Build history of the part. All positions in model axes, mm. Face numbers are marked on the shaded views. Give positions to 0.01 mm unless a question says otherwise; leave off trailing zeros. Order: outer loops, then holes, each group sorted by start corner. A loop starts at its lowest first (then second) coordinate and runs counter-clockwise, first axis right, second up. Notation, with made-up numbers: M -22,67.5 L -17,67.5 A9 ccw -17,77.5 Z; hole C 53,25 d5. An arc over 180 degrees is marked long. One line per item, written item: value.
from build123d import *

# Parameters (mm, degrees)
BOSS_EXTRUDE1_START      = -1
SKETCH1_W                = 40
SKETCH1_H                = 10
BOSS_EXTRUDE1_DEPTH      = 5
BOSS_EXTRUDE2_DEPTH      = 5
BOSS_EXTRUDE2_DEPTH_BACK = 5
SKETCH3_W                = 10
SKETCH3_H                = 10
BOSS_EXTRUDE3_DEPTH      = 5
FILLET1_R                = 3
FILLET2_R                = 3
FILLET3_R                = 0.5
FILLET4_R                = 10
CUT_EXTRUDE1_DEPTH       = 25.669870287
CUT_EXTRUDE1_DEPTH_BACK  = 25.669870287
SKETCH4_R                = 1.875
CUT_EXTRUDE2_START       = 5
SKETCH5_R                = 3.5
CUT_EXTRUDE2_DEPTH       = 10
SKETCH7_W                = 51.703075982
SKETCH7_H                = 23.04476915
CUT_EXTRUDE4_DEPTH       = 25.669870308


with BuildPart() as part:
    # Sketch1 → Boss-Extrude1 (new body)
    with BuildSketch(Plane(origin=(0, 0, 0), x_dir=(1, 0, 0), z_dir=(0, 1, 0)).offset(BOSS_EXTRUDE1_START)):
        Rectangle(SKETCH1_W, SKETCH1_H)
    extrude(amount=-BOSS_EXTRUDE1_DEPTH)

    # Fillet2
    fillet2_edges = [part.edges().sort_by_distance(p)[0] for p in [
        (20, -3.5, 5),
        (-20, -3.5, 5),
        (-20, -3.5, -5),
        (20, -3.5, -5),
    ]]
    fillet(fillet2_edges, radius=FILLET2_R)


with BuildPart() as body_2:
    # Sketch2 → Boss-Extrude2 (new, two sides: drawn at the far end of the back side and taken through both)
    with BuildSketch(Plane.XY.offset(-BOSS_EXTRUDE2_DEPTH_BACK)):
        with BuildLine():
            Line((-10.378945033, 0), (-4.733920151, 0))
            ThreePointArc((-4.733920151, 0), (0, 8.3), (4.733920151, 0))
            Line((4.733920151, 0), (10.378945033, 0))
            ThreePointArc((10.378945033, 0), (0, 13.55), (-10.378945033, 0))
        make_face()
    extrude(amount=BOSS_EXTRUDE2_DEPTH + BOSS_EXTRUDE2_DEPTH_BACK)

    # Sketch3 → Boss-Extrude3 (add)
    with BuildSketch(Plane(origin=(0, 0, 0), x_dir=(1, 0, 0), z_dir=(0, 1, 0))):
        with Locations((-15, 0)):
            Rectangle(SKETCH3_W, SKETCH3_H)
        with Locations((15, 0)):
            Rectangle(SKETCH3_W, SKETCH3_H)
    extrude(amount=BOSS_EXTRUDE3_DEPTH)

    # Fillet1
    fillet1_edges = [body_2.edges().sort_by_distance(p)[0] for p in [
        (-20, 2.5, -5),
        (-20, 2.5, 5),
        (20, 2.5, 5),
        (20, 2.5, -5),
    ]]
    fillet(fillet1_edges, radius=FILLET1_R)

    # Fillet3
    fillet3_edges = [body_2.edges().sort_by_distance(p)[0] for p in [
        (-4.733920151, 0, 0),
        (4.733920151, 0, 0),
    ]]
    fillet(fillet3_edges, radius=FILLET3_R)

    # Fillet4
    fillet4_edges = [body_2.edges().sort_by_distance(p)[0] for p in [
        (-10.522475944, 5, 0),
        (10.522475944, 5, 0),
    ]]
    fillet(fillet4_edges, radius=FILLET4_R)


with BuildPart() as cut_extrude1_tool:
    # Sketch4 → Cut-Extrude1 (new, two sides: drawn at the far end of the back side and taken through both)
    with BuildSketch(Plane(origin=(0, 0, 0), x_dir=(1, 0, 0), z_dir=(0, 1, 0)).offset(-CUT_EXTRUDE1_DEPTH_BACK)):
        with Locations(Location((-15.1, 0, 0), (0, 0, 206.04511236))):
            Circle(SKETCH4_R)
        with Locations(Location((15.1, 0, 0), (0, 0, 333.95488764))):
            Circle(SKETCH4_R)
    extrude(amount=CUT_EXTRUDE1_DEPTH + CUT_EXTRUDE1_DEPTH_BACK)


with BuildPart() as part_1:
    add(part.part)

    # Cut-Extrude1: cut by cut_extrude1_tool
    add(cut_extrude1_tool.part, mode=Mode.SUBTRACT)

    # Sketch7 → Cut-Extrude4 (cut, through all)
    with BuildSketch(Plane(origin=(0, 0, 0), x_dir=(1, 0, 0), z_dir=(0, 1, 0))):
        with Locations((-1.693322056, -1.721439234)):
            Rectangle(SKETCH7_W, SKETCH7_H)
    extrude(amount=-CUT_EXTRUDE4_DEPTH, mode=Mode.SUBTRACT)


with BuildPart() as body_2_1:
    add(body_2.part)

    # Cut-Extrude1: cut by cut_extrude1_tool
    add(cut_extrude1_tool.part, mode=Mode.SUBTRACT)

    # Sketch5 → Cut-Extrude2 (cut)
    with BuildSketch(Plane(origin=(0, 0, 0), x_dir=(1, 0, 0), z_dir=(0, 1, 0)).offset(CUT_EXTRUDE2_START)):
        with Locations((-15.1, 0)):
            Circle(SKETCH5_R)
        with Locations((15.1, 0)):
            Circle(SKETCH5_R)
    extrude(amount=CUT_EXTRUDE2_DEPTH, mode=Mode.SUBTRACT)


solid = body_2_1.part
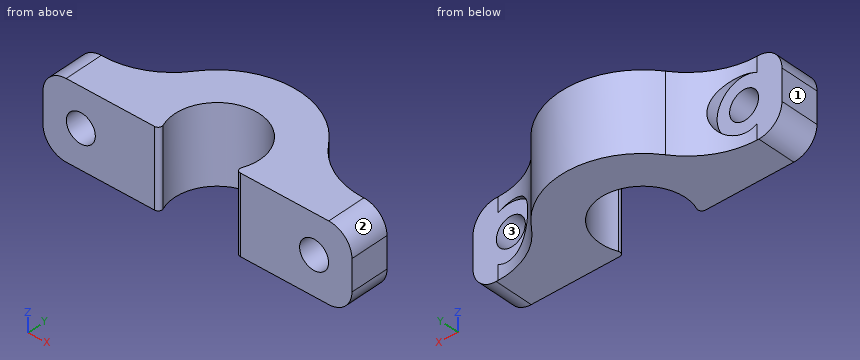
1) Saw through at C-C, the plane x = -15.5. Write the cut outline in (y, z).
Check values:
outline: M 0,-5 L 5.08,-5 L 5.08,-3.48 L 5,-3.48 L 5,-1.83 L 0,-1.83 Z; M 0,1.83 L 5,1.83 L 5,3.48 L 5.08,3.48 L 5.08,5 L 0,5 Z
2) Saw through at D-D, the plane y = 6. Write the cut outline in (x, z), then the cut area to 3 significant figures.
Check values:
outline: M -12.43,-5 L -4.47,-5 L -4.47,5 L -12.43,5 L -12.43,2.26 A3.5 cw -12.43,-2.26 Z; M 4.47,-5 L 12.43,-5 L 12.43,-2.26 A3.5 cw 12.43,2.26 L 12.43,5 L 4.47,5 Z
area: 154 mm^2
3) Saw through at B-B, the plane z = 1.5. Write the cut outline in (x, y) (3 decimals), then the cut area to 3 significant figures.
Check values:
outline: M -20,0 L -16.225,0 L -16.225,5 L -20,5 Z; M -13.975,0 L -5.542,0 A0.5 ccw -5.08,0.692 A5.5 cw long 5.08,0.692 A0.5 ccw 5.542,0 L 13.975,0 L 13.975,5 L 11.938,5 L 11.938,6.253 A10 cw 8.696,9.12 A10.75 ccw -8.696,9.12 A10 cw -11.938,6.253 L -11.938,5 L -13.975,5 Z; M 16.225,0 L 20,0 L 20,5 L 16.225,5 Z
area: 242 mm^2
4) Pin check, flat tips, straight feed: pin 1 (4 mm diameter, centred on x = -5, z = 2.5, fed in from +Y); pin 2 (1.5 mm diameter, centred on y = 9.5, z = -1.5, fed in from -X); pin 3 (1 mm diameter, centred on x = 3.5, z = 2.5, fed in from -Y). Stop position of each tip, or through.
Check values:
pin 1: y = 13.12
pin 2: x = -8.98
pin 3: y = 6.57
5) Saw through at A-A, the plane y = 2.8. Write the cut outline in (x, z) (3 decimals).
Check values:
outline: M -20,-2 A3 ccw -17,-5 L -5.5,-5 L -5.5,5 L -17,5 A3 ccw -20,2 Z; M 5.5,-5 L 17,-5 A3 ccw 20,-2 L 20,2 A3 ccw 17,5 L 5.5,5 Z; hole C -15.1,0 d3.75; hole C 15.1,0 d3.75
6) Drill centre lines: probe 1 along X at (y, z) = (2.85, 0) (3 decimals); probe 2 along Z at (x, y) = (-15.1, 2.55) (3 decimals); probe 3 along Y at (x, z) = (17, -2.25). Where is each one in solid material? Low to high. Write a range as from..to.
Check values:
probe 1: -20..-16.975, -13.225..-5.5, 5.5..13.225, 16.975..20
probe 2: -5..-1.875, 1.875..5
probe 3: 0..5
7) Mould opens along Z. For the marked faces 1, 2 and 3 say: released by +Z, released by -Z, zero draft, split by the parting line, or undercut.
Check values:
face 1: zero draft
face 2: released by +Z
face 3: undercut
